```python
from build123d import *

# Parameters (mm, degrees)
F0_R           = 7.5
F1_DEPTH       = 7.6
F1_DEPTH_BACK  = 17.3
F2_DEPTH       = 6.8
F4_DEPTH       = 4.4
F4_DEPTH_BACK  = 13.9
F6_W           = 51.2241850299
F6_H           = 71.6110350132
F7_DEPTH       = 5
F10_DEPTH      = 0.6
F11_W          = 51.2241850299
F11_H          = 21.4426852763
F12_DEPTH      = 4
F15_R          = 5
F16_DEPTH      = 25
F16_DEPTH_BACK = 25


with BuildPart() as f1:
    # F0 (on Top) → F1 (new body, two sides)
    with BuildSketch(Plane.XY) as f1_sk:
        with Locations((-21.15, 0)):
            Circle(F0_R)
    extrude(amount=F1_DEPTH)
    extrude(f1_sk.sketch, amount=-F1_DEPTH_BACK)


with BuildPart() as f1b:
    # F0 (on Top) → F1, piece 2 (new body, two sides)
    with BuildSketch(Plane.XY) as f1_2_sk:
        with Locations((21.15, 0)):
            Circle(F0_R)
    extrude(amount=F1_DEPTH)
    extrude(f1_2_sk.sketch, amount=-F1_DEPTH_BACK)


with BuildPart() as f2:
    # F0 (on Top) → F2 (new body)
    with BuildSketch(Plane.XY):
        Polygon((-6.5, 4.1165491707), (-6.5, 0), (-6.5, -4.1165491707), (0, -7.19), (6.5, -4.1165491707), (6.5, 0), (6.5, 4.1165491707), (0, 7.19), align=None)
    extrude(amount=-F2_DEPTH)


with BuildPart() as f4:
    # F3 (on Top) → F4 (new body, two sides)
    with BuildSketch(Plane.XY) as f4_sk:
        Polygon((-25.612092515, -21.15), (25.612092515, -21.15), (37.0736953387, 3.4294865757), (-37.0736953387, 3.4294865757), align=None)
    extrude(amount=F4_DEPTH)
    extrude(f4_sk.sketch, amount=-F4_DEPTH_BACK)

    # F5: cut F1, F2, F1b
    add(f1.part, mode=Mode.SUBTRACT)
    add(f2.part, mode=Mode.SUBTRACT)
    add(f1b.part, mode=Mode.SUBTRACT)

    # F6 (on face) → F7 (join)
    with BuildSketch(Plane.XZ.offset(21.15)):
        with Locations((0, 21.9055175066)):
            Rectangle(F6_W, F6_H)
    extrude(amount=F7_DEPTH)

    # F11 (on face) → F12 (join)
    with BuildSketch(Plane(origin=(0, -21.15, 0), x_dir=(-1, 0, 0), z_dir=(0, 1, 0))):
        with Locations((0, 46.9896923751)):
            Rectangle(F11_W, F11_H)
    extrude(amount=F12_DEPTH)


with BuildPart() as f10:
    # F9 (on offset) → F10 (new body)
    with BuildSketch(Plane(origin=(0, -20.55, 0), x_dir=(-1, 0, 0), z_dir=(0, 1, 0))):
        Polygon((-20, 58.7664473951), (-10.2, 40.7664473951), (20, 40.7664473951), (10.2, 58.7664473951), align=None)
    extrude(amount=-F10_DEPTH)


with BuildPart() as f4_1:
    add(f4.part)

    # F13: cut F10
    add(f10.part, mode=Mode.SUBTRACT)

    # F15 (on face) → F16 (cut, two sides)
    with BuildSketch(Plane(origin=(0, 0, -13.9), x_dir=(1, 0, 0), z_dir=(0, 0, -1))) as f16_sk:
        Circle(F15_R)
    extrude(amount=-F16_DEPTH, mode=Mode.SUBTRACT)
    extrude(f16_sk.sketch, amount=F16_DEPTH_BACK, mode=Mode.SUBTRACT)


solid = f4_1.part
```
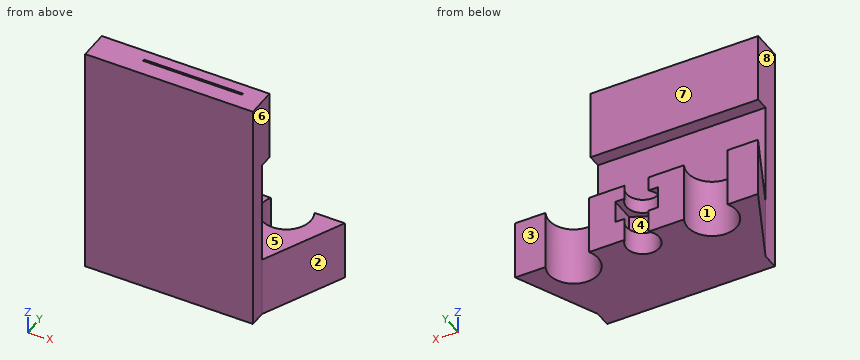
Read the model definition and answer for the solid it produces. Units are mm, in the model's axes. Face numbers are marked on the shaded views. A direction names the side the tool comes from. Coordinates: 2 decimals unless noted, no trailing zeros. Loops run counter-clockwise (first coordinate to the right, second up) from the corner with the lowest first, then second, coordinate; pieces in that order, holes last.
(1) A tool of negligible diameter and unlimited length cuts with its end or side. For the marked faces 4, 5, 6, 7 and 8, from which of +Z, -Z, +X, -X, +Y, -Y can it reach the whole face along a straight path? Write none if from no direction.
Solution:
face 4: +Y
face 5: +X, -X, +Y
face 6: +Z, +X, -Y
face 7: +Z, +X, -X, +Y
face 8: +Z, -X, -Y
(2) The part is cut by section C-C (z = -3). Determine the outline of the cut face in (x, y), and give its area (3 significant figures).
Solution:
outline: (-37.07, 3.43) - (-25.61, -21.15) - (-25.61, -26.15) - (25.61, -26.15) - (25.61, -21.15) - (37.07, 3.43) - (27.82, 3.43) arc R7.5 cw (long way) to (14.48, 3.43) - (6.5, 3.43) - (6.5, -4.12) - (0, -7.19) - (-6.5, -4.12) - (-6.5, 3.43) - (-14.48, 3.43) arc R7.5 cw (long way) to (-27.82, 3.43) - close
area: 1,400 mm2
(3) The part is cut by section D-D (y = -3). Determine the outline of the cut face in (x, z).
Solution:
outline: (-34.08, -13.9) - (-28.02, -13.9) - (-28.02, 4.4) - (-34.08, 4.4) - close; (-14.28, -13.9) - (-4, -13.9) - (-4, -6.8) - (-6.5, -6.8) - (-6.5, 0) - (-4, 0) - (-4, 4.4) - (-14.28, 4.4) - close; (4, -13.9) - (14.28, -13.9) - (14.28, 4.4) - (4, 4.4) - (4, 0) - (6.5, 0) - (6.5, -6.8) - (4, -6.8) - close; (28.02, -13.9) - (34.08, -13.9) - (34.08, 4.4) - (28.02, 4.4) - close
(4) The part is cut by section A-A (y = -18.25). Determine the outline of the cut face in (x, z).
Solution:
outline: (-26.96, -13.9) - (26.96, -13.9) - (26.96, 4.4) - (-26.96, 4.4) - close; (-25.61, 36.27) - (25.61, 36.27) - (25.61, 57.71) - (-25.61, 57.71) - close
(5) The mould has two halves that part along Y. Classify the marked faces 1, 2 and 3: released by +Y, released by -Y, zero draft, split by the parting line, or undercut.
Solution:
face 1: undercut
face 2: released by -Y
face 3: released by +Y
(6) Flat-ended cylindrical pins translate along their axes: pin 1 Ø4 at (x, z) = (-17, 1.5) entering from +Y; pin 2 Ø4.5 at (y, z) = (-21.5, 21.5) entering from -X; pin 3 Ø7.5 at (y, z) = (-1.5, -3) entering from +X. Find the tip coordinate at first contact, or state that the pin passes through.
Solution:
pin 1: stops at y = -4.29
pin 2: stops at x = -25.61
pin 3: stops at x = 36.52
(7) Consider line 1 along Y through (x, z) = (-8.5, 53); line 2 along X through (y, z) = (0, -3.75); line 3 along X through (y, z) = (0, -7.75). Determine where each line is inside the solid, lowest interval first.
Solution:
line 1: y = -26.15 to -21.15, -20.55 to -17.15
line 2: x = -35.47 to -28.65, -13.65 to -6.5, 6.5 to 13.65, 28.65 to 35.47
line 3: x = -35.47 to -28.65, -13.65 to -5, 5 to 13.65, 28.65 to 35.47
(8) The part is cut by section B-B (x = -21.15). Determine the outline of the cut face in (y, z), and give its area (3 significant figures).
Solution:
outline: (-26.15, -13.9) - (-7.5, -13.9) - (-7.5, 4.4) - (-21.15, 4.4) - (-21.15, 36.27) - (-17.15, 36.27) - (-17.15, 57.71) - (-26.15, 57.71) - close
area: 694 mm2
